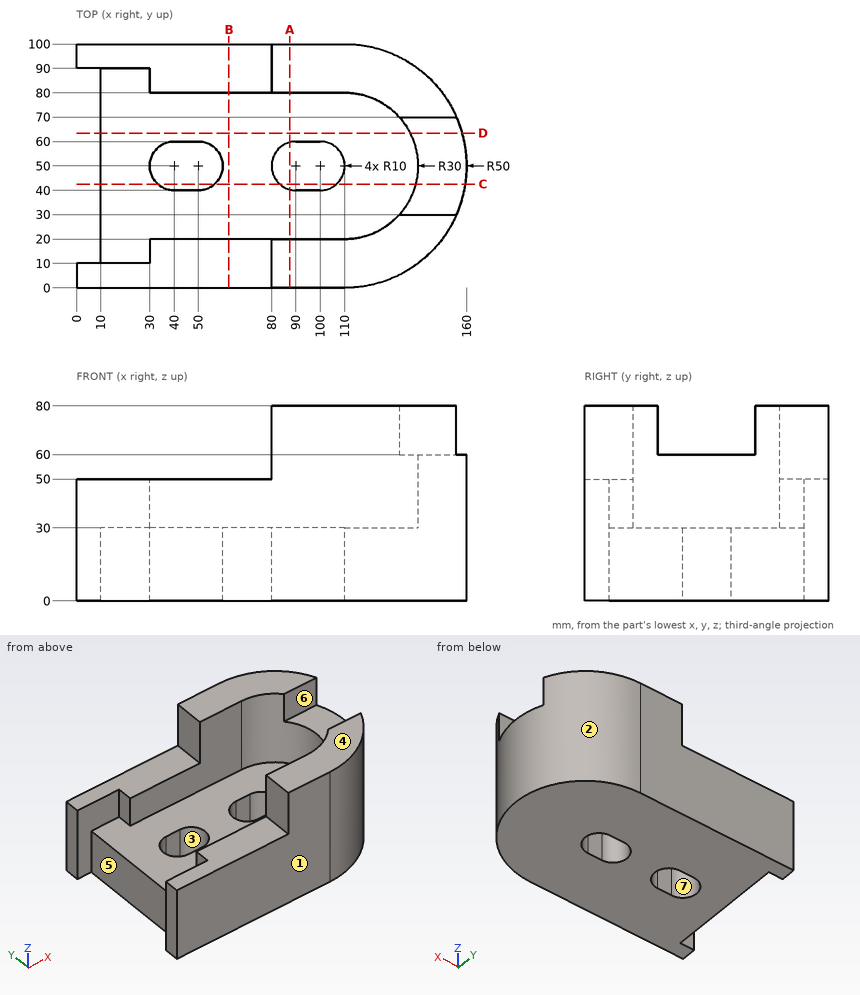
Source: three-view drawing plus pictorial views. Frame: mm from the lowest corner of the part. A direction names the side the tool comes from. Round coordinates to 2 decimals unless told otherwise and drop trailing zeros. Loops run counter-clockwise (first coordinate to the right, second up) from the corner with the lowest first, then second, coordinate; pieces in that order, holes last.
1. Section query B-B on x = 62.5. Output: boundary loops of the cut face in (y, z).
2. Mould query, pull axis Y, two halves, no side actions, for the marked faces 1, 2, 3 and 4. Classes: released by +Y, released by -Y, zero draft, split by the parting line, or undercut.
3. Contact query for flat-ended pins moving along their axis: pin 1 (22 mm diameter, centred on y = 94, z = 63.5, fed in from -X); pin 2 (10 mm diameter, centred on x = 148.5, z = 70.5, fed in from +Y); pin 3 (16 mm diameter, centred on x = 27.5, y = 7.5, fed in from +Z); pin 4 (5 mm diameter, centred on x = 95, z = 21, fed in from -Y). Output: stop coordinate, or through.
4. Access query for the marked faces 5, 6 and 7. Directions: +Z, -Z, +X, -X, +Y, -Y. A direction counts if a zero-diameter tool reaches every point of the face in a straight line with its end or side. Return the directions, or none.
5. Section query C-C on y = 42.5. Output: boundary loops of the cut face in (x, z).
6. Section query D-D on y = 63.5. Output: boundary loops of the cut face in (x, z).
7. Ray query, L1, parallel to Y at x = 42.5, z = 21.5; L2, parallel to X at y = 42, z = 17; L3, parallel to Y at x = 25.5, z = 48.5. Return the intervals inside material, ascending.
8. Section query A-A on x = 87.5. Output: boundary loops of the cut face in (y, z).
Answers below:
1. outline: (0, 0) - (100, 0) - (100, 50) - (80, 50) - (80, 30) - (20, 30) - (20, 50) - (0, 50) - close
2. face 1: released by -Y
2. face 2: split by the parting line
2. face 3: undercut
2. face 4: zero draft
3. pin 1: stops at x = 80
3. pin 2: stops at y = 87.12
3. pin 3: stops at z = 50
3. pin 4: stops at y = 0
4. face 5: +Z, -Z, -X
4. face 6: +Z, +X, -X
4. face 7: +Z, -Z
5. outline: (10, 0) - (33.39, 0) - (33.39, 30) - (10, 30) - close; (56.61, 0) - (83.39, 0) - (83.39, 30) - (56.61, 30) - close; (106.61, 0) - (159.43, 0) - (159.43, 60) - (139.05, 60) - (139.05, 30) - (106.61, 30) - close
6. outline: (10, 0) - (158.14, 0) - (158.14, 60) - (136.79, 60) - (136.79, 30) - (10, 30) - close
7. L1: y = 0 to 40, 60 to 100
7. L2: x = 10 to 34, 56 to 84, 106 to 159.36
7. L3: y = 0 to 10, 90 to 100
8. outline: (0, 0) - (40.32, 0) - (40.32, 30) - (20, 30) - (20, 80) - (0, 80) - close; (59.68, 0) - (100, 0) - (100, 80) - (80, 80) - (80, 30) - (59.68, 30) - close
